from build123d import *

# Parameters (mm, degrees)
SKETCH1_W               = 150
SKETCH1_H               = 160
BOSS_EXTRUDE1_DEPTH     = 20
CUT_EXTRUDE1_DEPTH      = 15
CUT_EXTRUDE1_DEPTH_BACK = 15
SKETCH2_W               = 60
SKETCH2_H               = 67.5
CUT_EXTRUDE6_DEPTH      = 10
CUT_EXTRUDE6_DEPTH_BACK = 0.1
REVOLVE2_ANGLE          = 180
REVOLVE3_ANGLE          = 180
REVOLVE4_ANGLE          = 180
REVOLVE5_ANGLE          = 180
REVOLVE6_ANGLE          = 180
REVOLVE7_ANGLE          = 180
REVOLVE8_ANGLE          = 180
REVOLVE9_ANGLE          = 180
REVOLVE10_ANGLE         = 180
REVOLVE11_ANGLE         = 180


with BuildPart() as part:
    # Sketch1 → Boss-Extrude1 (new body)
    with BuildSketch(Plane(origin=(0, 0, 0), x_dir=(1, 0, 0), z_dir=(0, 1, 0))):
        with Locations((0.216138329, 49.200288184)):
            Rectangle(SKETCH1_W, SKETCH1_H)
    extrude(amount=BOSS_EXTRUDE1_DEPTH)

    # Sketch2 → Cut-Extrude1 (cut, two sides: drawn at the far end of the back side and taken through both)
    with BuildSketch(Plane(origin=(0, 0, 0), x_dir=(1, 0, 0), z_dir=(0, 1, 0)).offset(-CUT_EXTRUDE1_DEPTH_BACK)):
        with Locations((-29.783861671, 62.950288184)):
            Rectangle(SKETCH2_W, SKETCH2_H)
    extrude(amount=CUT_EXTRUDE1_DEPTH + CUT_EXTRUDE1_DEPTH_BACK, mode=Mode.SUBTRACT)

    # Sketch3 → Cut-Revolve1 (revolve, cut)
    with BuildSketch(Plane(origin=(0, 0, 0), x_dir=(1, 0, 0), z_dir=(0, 1, 0))):
        Polygon((0.216138329, 96.700288184), (40.216138329, 95.450288184), (40.216138329, 89.200288184), (0.216138329, 89.200288184), align=None)
    revolve(axis=Axis((0.216138329, 0, -89.200288184), (1, 0, 0)), mode=Mode.SUBTRACT)

    # Sketch4 → Cut-Revolve2 (revolve, cut)
    with BuildSketch(Plane(origin=(0, 0, 0), x_dir=(1, 0, 0), z_dir=(0, 1, 0))):
        Polygon((0.216138329, 79.200288184), (60.216138329, 77.950288184), (60.216138329, 71.700288184), (0.216138329, 71.700288184), align=None)
    revolve(axis=Axis((94.987400497, 0, -71.700288184), (-1, 0, 0)), mode=Mode.SUBTRACT)

    # Sketch6 → Cut-Revolve3 (revolve, cut)
    with BuildSketch(Plane(origin=(0, 0, 0), x_dir=(1, 0, 0), z_dir=(0, 1, 0))):
        Polygon((0.216138329, 61.700288184), (60.216138329, 60.450288184), (60.216138329, 54.200288184), (0.216138329, 54.200288184), align=None)
    revolve(axis=Axis((60.216138329, 0, -54.200288184), (-1, 0, 0)), mode=Mode.SUBTRACT)

    # Sketch7 → Cut-Revolve4 (revolve, cut)
    with BuildSketch(Plane(origin=(0, 0, 0), x_dir=(1, 0, 0), z_dir=(0, 1, 0))):
        Polygon((0.216138329, 44.200288184), (60.216138329, 42.950288184), (60.216138329, 36.700288184), (0.216138329, 36.700288184), align=None)
    revolve(axis=Axis((60.216138329, 0, -36.700288184), (-1, 0, 0)), mode=Mode.SUBTRACT)

    # Sketch11 → Cut-Revolve5 (revolve, cut)
    with BuildSketch(Plane(origin=(0, 0, 0), x_dir=(1, 0, 0), z_dir=(0, 1, 0))):
        Polygon((-46.143861671, 29.200288184), (28.762467917, 1.110400544), (31.395894883, 8.132868943), (-24.783861671, 29.200288184), align=None)
    revolve(axis=Axis((28.762467917, 0, -1.110400544), (-0.9363291198500703, 0, -0.35112359550561795)), mode=Mode.SUBTRACT)

    # Sketch13 → Cut-Extrude6 (cut, two sides: drawn at the far end of the back side and taken through both)
    with BuildSketch(Plane(origin=(0, 0, 0), x_dir=(1, 0, 0), z_dir=(0, 1, 0)).offset(-CUT_EXTRUDE6_DEPTH_BACK)):
        Polygon((-30.050715604, 15.155351387), (-24.783861671, 29.200288184), (-46.143861671, 29.200288184), align=None)
    extrude(amount=CUT_EXTRUDE6_DEPTH + CUT_EXTRUDE6_DEPTH_BACK, mode=Mode.SUBTRACT)

    # Sketch15 → Revolve2 (revolve)
    with BuildSketch(Plane(origin=(0, 0, 0), x_dir=(1, 0, 0), z_dir=(0, 1, 0))):
        Polygon((50.216138329, 30.241954851), (37.716138329, 29.981538184), (37.716138329, 31.481538184), (50.216138329, 31.741954851), align=None)
    revolve(axis=Axis((60.216138329, 0, -36.700288184), (-1, 0, 0)), revolution_arc=REVOLVE2_ANGLE)

    # Sketch16 → Revolve3 (revolve)
    with BuildSketch(Plane(origin=(0, 0, 0), x_dir=(1, 0, 0), z_dir=(0, 1, 0))):
        Polygon((25.216138329, 29.721121518), (12.716138329, 29.460704851), (12.716138329, 30.960704851), (25.216138329, 31.221121518), align=None)
    revolve(axis=Axis((60.216138329, 0, -36.700288184), (-1, 0, 0)), revolution_arc=REVOLVE3_ANGLE)

    # Sketch17 → Revolve4 (revolve)
    with BuildSketch(Plane(origin=(0, 0, 0), x_dir=(1, 0, 0), z_dir=(0, 1, 0))):
        Polygon((50.216138329, 47.741954851), (50.216138329, 49.241954851), (37.716138329, 48.981538184), (37.716138329, 47.481538184), align=None)
    revolve(axis=Axis((60.216138329, 0, -54.200288184), (-1, 0, 0)), revolution_arc=REVOLVE4_ANGLE)

    # Sketch18 → Revolve5 (revolve)
    with BuildSketch(Plane(origin=(0, 0, 0), x_dir=(1, 0, 0), z_dir=(0, 1, 0))):
        Polygon((25.216138329, 47.221121518), (25.216138329, 48.721121518), (12.716138329, 48.460704851), (12.716138329, 46.960704851), align=None)
    revolve(axis=Axis((60.216138329, 0, -54.200288184), (-1, 0, 0)), revolution_arc=REVOLVE5_ANGLE)

    # Sketch19 → Revolve6 (revolve)
    with BuildSketch(Plane(origin=(0, 0, 0), x_dir=(1, 0, 0), z_dir=(0, 1, 0))):
        Polygon((50.216138329, 65.241954851), (50.216138329, 66.741954851), (37.716138329, 66.481538184), (37.716138329, 64.981538184), align=None)
    revolve(axis=Axis((60.216138329, 0, -71.700288184), (-1, 0, 0)), revolution_arc=REVOLVE6_ANGLE)

    # Sketch20 → Revolve7 (revolve)
    with BuildSketch(Plane(origin=(0, 0, 0), x_dir=(1, 0, 0), z_dir=(0, 1, 0))):
        Polygon((25.216138329, 66.221121518), (25.216138329, 64.721121518), (12.716138329, 64.460704851), (12.716138329, 65.960704851), align=None)
    revolve(axis=Axis((60.216138329, 0, -71.700288184), (-1, 0, 0)), revolution_arc=REVOLVE7_ANGLE)

    # Sketch21 → Revolve8 (revolve)
    with BuildSketch(Plane(origin=(0, 0, 0), x_dir=(1, 0, 0), z_dir=(0, 1, 0))):
        Polygon((32.716138329, 82.715913184), (32.716138329, 84.215913184), (23.341138329, 83.922944434), (23.341138329, 82.422944434), align=None)
    revolve(axis=Axis((40.216138329, 0, -89.200288184), (-1, 0, 0)), revolution_arc=REVOLVE8_ANGLE)

    # Sketch22 → Revolve9 (revolve)
    with BuildSketch(Plane(origin=(0, 0, 0), x_dir=(1, 0, 0), z_dir=(0, 1, 0))):
        Polygon((13.966138329, 82.129975684), (13.966138329, 83.629975684), (4.591138329, 83.337006934), (4.591138329, 81.837006934), align=None)
    revolve(axis=Axis((40.216138329, 0, -89.200288184), (-1, 0, 0)), revolution_arc=REVOLVE9_ANGLE)

    # Sketch23 → Revolve10 (revolve)
    with BuildSketch(Plane(origin=(0, 0, 0), x_dir=(1, 0, 0), z_dir=(0, 1, 0))):
        Polygon((17.292435145, -0.99633822), (16.765749752, -2.4008319), (5.061635754, 1.988213044), (5.588321147, 3.392706724), align=None)
    revolve(axis=Axis((28.762467917, 0, -1.110400544), (-0.9363291198500702, 0, -0.35112359550561806)), revolution_arc=REVOLVE10_ANGLE)

    # Sketch25 → Revolve11 (revolve)
    with BuildSketch(Plane(origin=(0, 0, 0), x_dir=(1, 0, 0), z_dir=(0, 1, 0))):
        Polygon((-6.115792851, 7.781751668), (-6.642478245, 6.377257988), (-18.346592243, 10.766302932), (-17.819906849, 12.170796611), align=None)
    revolve(axis=Axis((28.762467917, 0, -1.110400544), (-0.9363291198500703, 0, -0.351123595505618)), revolution_arc=REVOLVE11_ANGLE)


solid = part.part
Check sheet for the modelled part. Datum: model origin and axes. Units: mm. A direction names the side the tool comes from. Round coordinates to 2 decimals unless told otherwise and drop trailing zeros. One line per item, written item: value. Start each with the question number.
1. Scan lines: line 1 along Z through (x, y) = (33, 2.75); line 2 along Z through (x, y) = (-38, 11); line 3 along X through (y, z) = (3, -55.5). Record each from-to range of solid material in increasing order.
2. Access from +Z, -Z, +X, -X, +Y, -Y to the whole of each face (thin tool, end or side, straight path). Record for faces 1 (the flat face through (7.51, 6.27, -8.52)), 2 (the flat face through (-1, 10, -129.2)).
3. Release check for a two-part mould opening along X. For faces 3 (the flat face through (50.216, 5.2, -72.2)), 4 (the flat face through (16, 0, -15)) record: released by +X, released by -X, zero draft, split by the parting line, or undercut.
4. Gauge pin test, flat ends, axial feed: P1, Ø6, axis at x = 30, z = -69, coming from the -Y side; P2, Ø11, axis at x = -30.5, z = -25, coming from the -Y side. Record the tip position at first contact, or that the pin passes through.
Results found:
1. line 1: -129.2 to -95.06, -83.34 to -77.94, -65.46 to -60.44, -47.96 to -42.94, -30.46 to 30.8
1. line 2: -129.2 to -96.7, -29.2 to 30.8
1. line 3: -74.78 to -59.78, 60.22 to 75.22
2. face 1: -Y
2. face 2: -Z, +X, -X, +Y, -Y
3. face 3: undercut
3. face 4: zero draft
4. P1: y = 3.85
4. P2: y = 5.14
